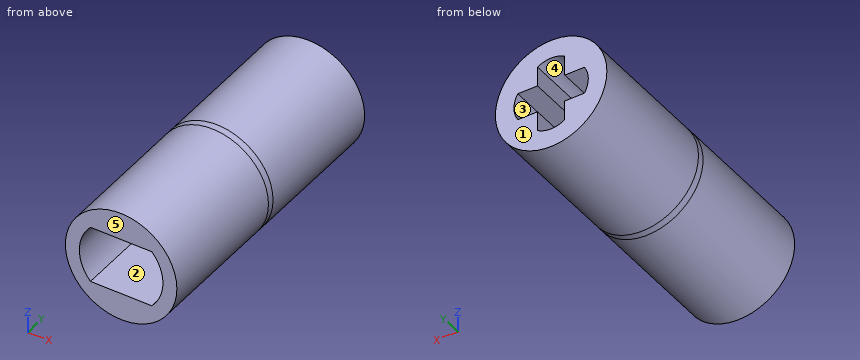
Autodesk Inventor part; units mm, degrees
ref_plane "YZ Plane" through (0, 0, 0) normal (1, 0, 0) x (0, 1, 0)
ref_plane "XZ Plane" through (0, 0, 0) normal (0, 1, 0) x (-1, 0, 0)
ref_plane "XY Plane" through (0, 0, 0) normal (0, 0, 1) x (1, 0, 0)
sketch "Sketch3" plane through (0, 0, 0) normal (0, 1, 0) x (-1, 0, 0)
  line L0 (2.3926, -0.9756) -> (2.3926, 0.9756)
  line L1 (2.3926, 0.9756) -> (0.9755, 0.9755)
  line L2 (0.9755, 0.9755) -> (0.9754, 2.3926)
  line L3 (0.9754, 2.3926) -> (-0.9756, 2.3926)
  arc A0 (0.9754, 2.3926) -> (-0.9756, 2.3926) centre (0, 0.8054) ccw
  arc A1 (2.3926, -0.9756) -> (2.3926, 0.9756) centre (0.8054, 0) ccw
  line L4 (2.3926, -0.9756) -> (0.9755, -0.9756)
  line L5 (0.9755, -0.9756) -> (0.9756, -2.3926)
  line L6 (0.9756, -2.3926) -> (-0.9755, -2.3926)
  arc A2 (-0.9755, -2.3926) -> (0.9756, -2.3926) centre (0, -0.8054) ccw
  line L7 (-0.9756, 2.3926) -> (-0.9756, 0.9756)
  line L8 (-0.9755, -2.3926) -> (-0.9756, -0.9755)
  line L9 (-0.9756, 0.9756) -> (-2.3926, 0.9756)
  line L10 (-2.3926, 0.9756) -> (-2.3925, -0.9755)
  line L11 (-2.3925, -0.9755) -> (-0.9756, -0.9755)
  arc A3 (-2.3926, 0.9756) -> (-2.3925, -0.9755) centre (-0.8054, 0) ccw
  circle A4 centre (0, 0) radius 4
  dimension "d23" = 1.951
  dimension "d24" = 1.9511
  dimension "d25" = 0.9756
  dimension "d28" = 1.4171
  dimension "d29" = 1.417
  dimension "d30" = 2.5838
  dimension "d31" = 1.863
  dimension "d32" = 1.863
  dimension "d33" = 1.417
  dimension "d34" = 1.9511
  dimension "d35" = 1.863
  dimension "d36" = 1.417
  dimension "d37" = 2.5838
  dimension "d38" = 1.9511
  dimension "d39" = 1.863
  dimension "d40" = 2.3925
  dimension "d41" = 2.3925
  dimension "d42" = 1.417
  dimension "d43" = 1.417
  dimension "d44" = 8
extrude "Extrusion1" add sketch "Sketch3" along normal blind 10
sketch "Sketch4" plane through (0, 0, 0) normal (0, -1, 0) x (1, 0, 0)
  circle A0 centre (0, 0) radius 4
extrude "Extrusion2" add sketch "Sketch4" along normal blind 0.5
sketch "Sketch5" plane through (0, -0.5, 0) normal (0, -1, 0) x (1, 0, 0)
  circle A0 centre (0, 0) radius 2.999
  line L0 (-0.0001, 2.0364) -> (-2.2016, 2.0364)
  line L1 (-0.9754, 2.3926) -> (-0.9755, 0.9755)
  line L2 (-0.0001, 2.0364) -> (2.2016, 2.0364)
  line L3 (-0.0001, -2.0369) -> (-2.2012, -2.0369)
  line L4 (-0.9755, -0.9756) -> (-0.9756, -2.3926)
  line L5 (-0.0001, -2.0369) -> (2.2012, -2.0369)
  circle A1 centre (0, 0) radius 4
  dimension "d49" = 5.998
  dimension "d50" = 2.0364
  dimension "d51" = 2.0369
  dimension "d52" = 2.2015
  dimension "d53" = 2.2012
  dimension "d56" = 8
extrude "Extrusion3" add sketch "Sketch5" along normal blind 10 contours L2 L0 A0 | A0 L3 L5 | A1
properties part number "motor_adapt"
The model under review builds one solid part; all positions refer to its coordinate system, in mm. Face numbers are marked on the shaded views. A direction names the side the tool comes from. Give positions to 0.01 mm unless a question says otherwise; leave off trailing zeros. Loops run counter-clockwise (first coordinate to the right, second up) from the corner with the lowest first, then second, coordinate; pieces in that order, holes last. Notation, with made-up numbers: (85, -22.75) -> (109, -22.75) arc R25 ccw to (109, 13.25) -> close; hole circle Ø11 at (-16, -4.75). An arc over 180 degrees is marked (long way). Put each result on its own line as item: value. Start each with the question number.
1. Wall thickness on probe 1 along Z at (x, y) = (0, -1); probe 2 along Z at (x, y) = (0, 1.5); probe 3 along X at (y, z) = (3.5, 1.75): over which ranges is each line inside the solid? List them lowest first.
2. For the marked faces 1, 2 and 3, list the 3-axis set-ups (+Z, -Z, +X, -X, +Y, -Y) from which the entire face can be reached by the end or side of a thin tool; tool diameter is ignored.
3. We need section B-B on x = 0. State the section outline as (y, z) points, then the cut area to 3 significant figures.
4. Mouldability with a two-part tool opening along Z and no side actions: class the marked faces 4 and 5 as released by +Z, released by -Z, zero draft, split by the parting line, or undercut.
5. We need section A-A on z = 0. State the section outline as (x, y) points, then the cut area to 3 significant figures.
6. Clearance check with flat-ended pins moving along their axes: P1, Ø0.7, axis at x = -1.5, y = 3, coming from the +Z side; P2, Ø1.6, axis at x = 1.5, y = 7, coming from the -Z side; P3, Ø0.7, axis at y = 3.5, z = -1.5, coming from the +X side. State where each tip first meets the part, or that it passes through.
7. We need section C-C on y = -3.5. State the section outline as (x, z) points, then the cut area to 3 significant figures.
Determined:
1. probe 1: -4 to -2.04, 2.04 to 4
1. probe 2: -4 to -2.67, 2.67 to 4
1. probe 3: -3.6 to -0.98, 0.98 to 3.6
2. face 1: +Z, -Z, +X, -X, +Y
2. face 2: -Y
2. face 3: +Y
3. outline: (-10.5, -4) -> (10, -4) -> (10, -2.67) -> (0, -2.67) -> (0, 2.67) -> (10, 2.67) -> (10, 4) -> (-10.5, 4) -> (-10.5, 2.04) -> (-0.5, 2.04) -> (-0.5, -2.04) -> (-10.5, -2.04) -> close
3. area: 69.9 mm^2
4. face 4: undercut
4. face 5: zero draft
5. outline: (-4, -10.5) -> (-3, -10.5) -> (-3, -0.5) -> (3, -0.5) -> (3, -10.5) -> (4, -10.5) -> (4, 10) -> (2.67, 10) -> (2.67, 0) -> (-2.67, 0) -> (-2.67, 10) -> (-4, 10) -> close
5. area: 50.7 mm^2
6. P1: z = 3.83
6. P2: z = -3.94
6. P3: x = 3.83
7. outline: circle Ø8 at (0, 0); hole (-2.2, -2.04) -> (2.2, -2.04) arc R3 ccw to (2.2, 2.04) -> (-2.2, 2.04) arc R3 ccw to start
7. area: 27.9 mm^2
